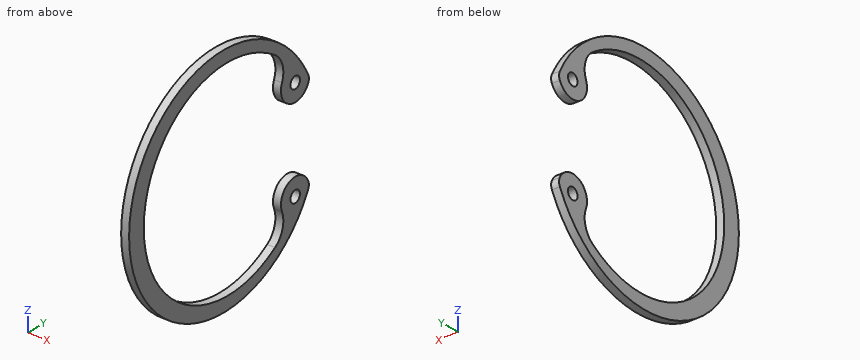
```python
from build123d import *

# Parameters (mm, degrees)
SKETCH_1_R      = 1.25
EXTRUDE_1_DEPTH = 1.7


with BuildPart() as part:
    # Эскиз1 → Бобышка-Вытянуть1 (new body)
    with BuildSketch(Plane(origin=(0, 0, 0), x_dir=(0, 0, -1), z_dir=(1, 0, 0))):
        with BuildLine():
            ThreePointArc((-10.884792801, 22.227995539), (0, -24.75), (10.884792801, 22.227995539))
            ThreePointArc((10.884792801, 22.227995539), (10.021540765, 22.431727234), (9.155077538, 22.242116696))
            ThreePointArc((9.155077538, 22.242116696), (7.311355918, 17.353467341), (12.145333072, 15.370825971))
            ThreePointArc((12.145333072, 15.370825971), (15.454308904, 15.51747296), (18.128902676, 13.563662694))
            ThreePointArc((18.128902676, 13.563662694), (0, -20.9), (-18.128902676, 13.563662694))
            ThreePointArc((-18.128902676, 13.563662694), (-15.454308904, 15.51747296), (-12.145333072, 15.370825971))
            ThreePointArc((-12.145333072, 15.370825971), (-7.311355918, 17.353467341), (-9.155077538, 22.242116696))
            ThreePointArc((-9.155077538, 22.242116696), (-10.021540765, 22.431727234), (-10.884792801, 22.227995539))
        make_face()
        with Locations((10.748404378, 18.84920571)):
            Circle(SKETCH_1_R, mode=Mode.SUBTRACT)
        with Locations((-10.748404378, 18.84920571)):
            Circle(SKETCH_1_R, mode=Mode.SUBTRACT)
    extrude(amount=EXTRUDE_1_DEPTH)


solid = part.part
```
Input: part model. Units: mm. Frame: model coordinates. Give positions to 0.01 mm unless a question says otherwise; leave off trailing zeros. Order: outer loops, then holes, each group sorted by start corner. A loop starts at its lowest first (then second) coordinate and runs counter-clockwise, first axis right, second up. Notation, with made-up numbers: (35.5, -5.5) - (41.5, -5.5) arc R18 cw to (41.5, 11.5) - close; hole circle Ø4 at (-24.5, 0.5). An arc over 180 degrees is marked (long way). One line per item, written item: value.
1. Line query: probe 1 along Y at (x, z) = (1.15, 0); probe 2 along Z at (x, y) = (0.95, -3); probe 3 along Z at (x, y) = (1.55, 6). Output: solid intervals per line, ascending.
Determined:
probe 1: -24.75 to -20.9
probe 2: -24.57 to -21.61, 21.61 to 24.57
probe 3: -24.01 to -21.45, 21.45 to 24.01
2. Cut plane D-D, the plane z = 0. Output: boundary loops of the cut face in (x, y), and give its area (4 significant figures).
Determined:
outline: (0, -24.75) - (1.7, -24.75) - (1.7, -20.9) - (0, -20.9) - close
area: 6.545 mm2
3. Cut plane B-B, the plane y = -13. Output: boundary loops of the cut face in (x, z), and give its area (3 significant figures).
Determined:
outline: (0, -21.06) - (1.7, -21.06) - (1.7, -16.89) - (0, -16.89) - close; (0, 16.89) - (1.7, 16.89) - (1.7, 21.06) - (0, 21.06) - close
area: 14.2 mm2
4. Cut plane A-A, the plane z = -17. Output: boundary loops of the cut face in (x, y).
Determined:
outline: (0, -17.99) - (1.7, -17.99) - (1.7, -12.86) - (0, -12.86) - close; (0, 14.74) - (1.7, 14.74) - (1.7, 17.99) - (0, 17.99) - close
5. Cut plane C-C, the plane x = 1.1. Output: boundary loops of the cut face in (y, z), and give its area (3 significant figures).
Determined:
outline: (13.56, -18.13) arc R22 cw (long way) to (13.56, 18.13) arc R5 cw to (15.37, 12.15) arc R3.75 ccw to (22.24, 9.16) arc R2 ccw to (22.23, 10.88) arc R24.75 ccw (long way) to (22.23, -10.88) arc R2 ccw to (22.24, -9.16) arc R3.75 ccw to (15.37, -12.15) arc R5 cw to start; hole circle Ø2.5 at (18.85, -10.75); hole circle Ø2.5 at (18.85, 10.75)
area: 433 mm2
